The listing builds one solid part. Answer for the finished solid, in the listing's coordinates (mm). Face numbers are marked on the shaded views. A direction names the side the tool comes from. Round coordinates to 2 decimals unless told otherwise and drop trailing zeros. Write each loop counter-clockwise with the first axis right and the second up, starting at its lowest first coordinate (ties: lowest second). Pieces come first, ordered by that corner, then holes.
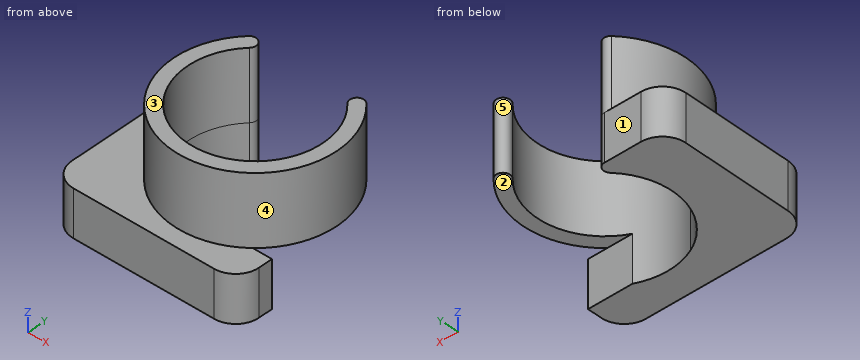
from build123d import *

# Parameters (mm, degrees)
BOSS_EXTRUDE1_START = 10
BOSS_EXTRUDE1_DEPTH = 15
BOSS_EXTRUDE3_DEPTH = 10
FILLET1_R           = 5
BOSS_EXTRUDE4_START = 10
BOSS_EXTRUDE4_DEPTH = 10


with BuildPart() as part:
    # Sketch1 → Boss-Extrude1 (new body)
    with BuildSketch(Plane.XY.offset(BOSS_EXTRUDE1_START)):
        with BuildLine():
            ThreePointArc((8.488266962, -3.382949128), (-2.000000007, -27.895254363), (-12.488266953, -3.382949118))
            ThreePointArc((-12.488266953, -3.382949118), (-12.537504406, -1.262200246), (-14.658253277, -1.311437749))
            ThreePointArc((-14.658253277, -1.311437749), (-1.999999957, -30.895254363), (10.658253217, -1.311437686))
            ThreePointArc((10.658253217, -1.311437686), (8.53750437, -1.262200281), (8.488266962, -3.382949128))
        make_face()
    extrude(amount=BOSS_EXTRUDE1_DEPTH)

    # Sketch2 → Boss-Extrude3 (add)
    with BuildSketch(Plane.XY):
        with BuildLine():
            ThreePointArc((-12.488266958, -3.382949123), (-12.194196355, -1.757122894), (-13.573260086, -0.847193408))
            ThreePointArc((-13.573260086, -0.847193408), (-14.163330605, -0.968129672), (-14.658253225, -1.311437694))
            ThreePointArc((-14.658253225, -1.311437694), (-19.372506678, -15.503811146), (-11.4, -28.156351884))
            Line((-11.4, -28.156351884), (-11.4, -26.495254363))
            Line((-11.4, -26.495254363), (-11.4, -24.435634792))
            ThreePointArc((-11.4, -24.435634792), (-16.480665872, -14.143796874), (-12.488266958, -3.382949123))
        make_face()
        with BuildLine():
            ThreePointArc((-14.658253225, -1.311437694), (-14.163330605, -0.968129672), (-13.573260086, -0.847193408))
            Line((-13.573260086, -0.847193408), (-26.4, -0.847193408))
            Line((-26.4, -0.847193408), (-26.4, -34.495254363))
            Line((-26.4, -34.495254363), (-11.4, -34.495254363))
            Line((-11.4, -34.495254363), (-11.4, -28.156351884))
            ThreePointArc((-11.4, -28.156351884), (-19.372506678, -15.503811146), (-14.658253225, -1.311437694))
        make_face()
        with BuildLine():
            ThreePointArc((9.603447763, -26.495254363), (-0.620287438, -30.840780817), (-11.4, -28.156351884))
            Line((-11.4, -28.156351884), (-11.4, -34.495254363))
            Line((-11.4, -34.495254363), (13.729379502, -34.495254363))
            Line((13.729379502, -34.495254363), (13.729379502, -26.495254363))
            Line((13.729379502, -26.495254363), (9.603447763, -26.495254363))
        make_face()
        with BuildLine():
            Line((-8.216108107, -26.495254363), (-11.4, -26.495254363))
            Line((-11.4, -26.495254363), (-11.4, -28.156351884))
            ThreePointArc((-11.4, -28.156351884), (-0.620287438, -30.840780817), (9.603447763, -26.495254363))
            Line((9.603447763, -26.495254363), (4.216108107, -26.495254363))
            ThreePointArc((4.216108107, -26.495254363), (-2, -27.895254363), (-8.216108107, -26.495254363))
        make_face()
    extrude(amount=BOSS_EXTRUDE3_DEPTH)

    # Fillet1
    fillet1_edges = [part.edges().sort_by_distance(p)[0] for p in [
        (-26.4, -34.495254363, 5),
        (13.729379502, -34.495254363, 5),
        (-26.4, -0.847193408, 5),
    ]]
    fillet(fillet1_edges, radius=FILLET1_R)

    # Sketch4 → Boss-Extrude4 (add)
    with BuildSketch(Plane(origin=(0, 0, 10), x_dir=(-1, 0, 0), z_dir=(0, 0, -1)).offset(BOSS_EXTRUDE4_START)):
        with BuildLine():
            Line((8.216108107, -26.495254363), (11.4, -26.495254363))
            Line((11.4, -26.495254363), (11.4, -24.435634792))
            ThreePointArc((11.4, -24.435634792), (9.875672435, -25.569973403), (8.216108107, -26.495254363))
        make_face()
    extrude(amount=-BOSS_EXTRUDE4_DEPTH)


solid = part.part
1. For a pull along X with two mould halves and no side action, classify the marked faces 3, 4 and 5 as released by +X, released by -X, zero draft, split by the parting line, or undercut.
Geometry says:
face 3: zero draft
face 4: split by the parting line
face 5: undercut
2. Straight lines are drawn through the part: line 1 along Y through (x, z) = (-2, 17); line 2 along X through (y, z) = (-24.5, 23); line 3 along Z through (x, y) = (-21.5, -10). For each, find the intervals that lie inside material, in ascending order.
Geometry says:
line 1: y = -30.9 to -27.9
line 2: x = -15.53 to -11.32, 7.32 to 11.53
line 3: z = 0 to 10
3. A tool of negligible diameter and unlimited length cuts with its end or side. For the marked faces 1 and 2, from which of +Z, -Z, +X, -X, +Y, -Y can it reach the whole face along a straight path? Write none if from no direction.
Geometry says:
face 1: +Z, -Z, +X, -X, +Y
face 2: -Z, +X, +Y
4. Section B-B on x = 11.5 is taken. Determine the outline of the cut face in (y, z).
Geometry says:
outline: (-33.66, 0) - (-26.5, 0) - (-26.5, 10) - (-33.66, 10) - close; (-24.53, 10) - (-18.69, 10) - (-18.69, 25) - (-24.53, 25) - close; (-8.1, 10) - (-2.26, 10) - (-2.26, 25) - (-8.1, 25) - close
5. Given pin 1 (17 mm diameter, centred on x = 1, y = -19, fed in from +Z); pin 2 (8 mm diameter, centred on x = -15.5, z = 21, fed in from -Y); pin 3 (8 mm diameter, centred on y = -8, z = 19, fed in from -X); pin 4 (12.5 mm diameter, centred on x = 9, y = -12.5, fed in from -Z), each flat-ended and moving along its own axis, determine where each tip first touches the part or whether it passes through.
Geometry says:
pin 1: stops at z = 25
pin 2: stops at y = -28.09
pin 3: stops at x = -19.44
pin 4: stops at z = 10
6. Section C-C on z = 3 is taken. Determine the outline of the cut face in (x, y), plus the area to 3 significant figures.
Geometry says:
outline: (-26.4, -29.5) arc R5 ccw to (-21.4, -34.5) - (8.73, -34.5) arc R5 ccw to (13.73, -29.5) - (13.73, -26.5) - (4.22, -26.5) arc R14.5 cw to (-12.49, -3.38) arc R1.5 ccw to (-13.57, -0.85) - (-21.4, -0.85) arc R5 ccw to (-26.4, -5.85) - close
area: 601 mm2
7. Section A-A on y = -11.5 is taken. Determine the outline of the cut face in (x, z), plus the area to 3 significant figures.
Geometry says:
outline: (-26.4, 0) - (-16.38, 0) - (-16.38, 25) - (-19.4, 25) - (-19.4, 10) - (-26.4, 10) - close; (12.38, 10) - (15.4, 10) - (15.4, 25) - (12.38, 25) - close
area: 191 mm2
8. Section D-D on x = -2 is taken. Determine the outline of the cut face in (y, z).
Geometry says:
outline: (-34.5, 0) - (-27.9, 0) - (-27.9, 25) - (-30.9, 25) - (-30.9, 10) - (-34.5, 10) - close
